Read the model definition and answer for the solid it produces. Units are mm, in the model's axes. Face numbers are marked on the shaded views. A direction names the side the tool comes from. Give positions to 0.01 mm unless a question says otherwise; leave off trailing zeros. Order: outer loops, then holes, each group sorted by start corner. A loop starts at its lowest first (then second) coordinate and runs counter-clockwise, first axis right, second up.
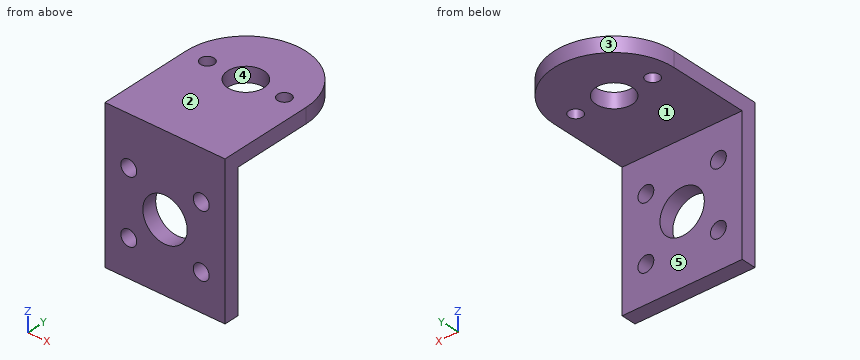
```python
from build123d import *

# Parameters (mm, degrees)
SKETCH_1_R          = 4
SKETCH_1_R_2        = 1.5
EXTRUDE_1_DEPTH     = 3.3
SKETCH_2_W          = 26.5
SKETCH_2_H          = 3.3
EXTRUDE_2_DEPTH     = 29.7
SKETCH_3_R          = 4.9
SKETCH_3_R_2        = 1.75
CUT_EXTRUDE_1_DEPTH = 3.3


with BuildPart() as part:
    # 草图1 → 凸台-拉伸1 (new body)
    with BuildSketch(Plane.XY):
        with BuildLine():
            Line((-13.25, 0), (-13.25, -20.75))
            Line((-13.25, -20.75), (13.25, -20.75))
            Line((13.25, -20.75), (13.25, 0))
            ThreePointArc((13.25, 0), (0, 13.25), (-13.25, 0))
        make_face()
        Circle(SKETCH_1_R, mode=Mode.SUBTRACT)
        with Locations((-8.5, 0)):
            Circle(SKETCH_1_R_2, mode=Mode.SUBTRACT)
        with Locations(Location((8.5, 0, 0), (0, 0, 180))):
            Circle(SKETCH_1_R_2, mode=Mode.SUBTRACT)
    extrude(amount=EXTRUDE_1_DEPTH)

    # 草图2 → 凸台-拉伸2 (add)
    with BuildSketch(Plane.XY):
        with Locations((0, -19.1)):
            Rectangle(SKETCH_2_W, SKETCH_2_H)
    extrude(amount=-EXTRUDE_2_DEPTH)

    # 草图3 → 切除-拉伸1 (cut)
    with BuildSketch(Plane(origin=(0, -17.45, 0), x_dir=(1, 0, 0), z_dir=(0, 1, 0))):
        with Locations(Location((0, 14.5, 0), (0, 0, 180))):
            Circle(SKETCH_3_R)
        with Locations(Location((-8, 21.55, 0), (0, 0, 180))):
            Circle(SKETCH_3_R_2)
        with Locations(Location((-8, 7.55, 0), (0, 0, 180))):
            Circle(SKETCH_3_R_2)
        with Locations(Location((8, 7.55, 0), (0, 0, 270))):
            Circle(SKETCH_3_R_2)
        with Locations(Location((8, 21.55, 0), (0, 0, 270))):
            Circle(SKETCH_3_R_2)
    extrude(amount=-CUT_EXTRUDE_1_DEPTH, mode=Mode.SUBTRACT)


solid = part.part
```
1) The part is cut by section C-C on z = 0.5. Determine the outline of the cut face in (x, y), and give its area (3 significant figures).
Final values:
outline: (-13.25, -20.75) - (13.25, -20.75) - (13.25, 0) arc R13.25 ccw to (-13.25, 0) - close; hole circle Ø3 at (-8.5, 0); hole circle Ø8 at (0, 0); hole circle Ø3 at (8.5, 0)
area: 761 mm2
2) Consider L1, parallel to Z at x = -8, y = -18.4; L2, parallel to X at y = -18, z = -21.5; L3, parallel to Z at x = 0, y = -19.8. Determine where each line is inside the solid, lowest interval first.
Final values:
L1: z = -29.7 to -23.3, -19.8 to -9.3, -5.8 to 3.3
L2: x = -13.25 to -9.75, -6.25 to 6.25, 9.75 to 13.25
L3: z = -29.7 to -19.4, -9.6 to 3.3
3) The part is cut by section B-B on x = 0. Determine the outline of the cut face in (y, z), and give its area (3 significant figures).
Final values:
outline: (-20.75, -29.7) - (-17.45, -29.7) - (-17.45, -19.4) - (-20.75, -19.4) - close; (-20.75, -9.6) - (-17.45, -9.6) - (-17.45, 0) - (-4, 0) - (-4, 3.3) - (-20.75, 3.3) - close; (4, 0) - (13.25, 0) - (13.25, 3.3) - (4, 3.3) - close
area: 151 mm2
4) A tool of negligible diameter and unlimited length cuts with its end or side. For the marked faces 1 and 2, from which of +Z, -Z, +X, -X, +Y, -Y can it reach the whole face along a straight path? Write none if from no direction.
Final values:
face 1: -Z, +X, -X, +Y
face 2: +Z, +X, -X, +Y, -Y
5) For a pull along X with two mould halves and no side action, classify the marked faces 3, 4 and 5 as released by +X, released by -X, zero draft, split by the parting line, or undercut.
Final values:
face 3: split by the parting line
face 4: undercut
face 5: zero draft
6) Given pin 1 (1.5 mm diameter, centred on x = -9.5, z = -5, fed in from +Y); pin 2 (12 mm diameter, centred on x = 9.5, z = -21, fed in from -Y); pin 3 (13 mm diameter, centred on x = -0.5, y = 1, fed in from -Z); pin 4 (1.8 mm diameter, centred on x = -8.5, y = 0, fed in from -Z), each flat-ended and moving along its own axis, determine where each tip first touches the part or whether it passes through.
Final values:
pin 1: stops at y = -17.45
pin 2: stops at y = -20.75
pin 3: stops at z = 0
pin 4: passes through
7) The part is cut by section A-A on z = -7.55. Determine the outline of the cut face in (x, y), and give its area (4 significant figures).
Final values:
outline: (-13.25, -20.75) - (-9.75, -20.75) - (-9.75, -17.45) - (-13.25, -17.45) - close; (-6.25, -20.75) - (6.25, -20.75) - (6.25, -17.45) - (-6.25, -17.45) - close; (9.75, -20.75) - (13.25, -20.75) - (13.25, -17.45) - (9.75, -17.45) - close
area: 64.35 mm2
8) The part is cut by section D-D on x = 8.5. Determine the outline of the cut face in (y, z).
Final values:
outline: (-20.75, -29.7) - (-17.45, -29.7) - (-17.45, -23.23) - (-20.75, -23.23) - close; (-20.75, -19.87) - (-17.45, -19.87) - (-17.45, -9.23) - (-20.75, -9.23) - close; (-20.75, -5.87) - (-17.45, -5.87) - (-17.45, 0) - (-1.5, 0) - (-1.5, 3.3) - (-20.75, 3.3) - close; (1.5, 0) - (10.16, 0) - (10.16, 3.3) - (1.5, 3.3) - close
